Verification items for this drawing (mm, ordinates from the low corner). Coordinates: 2 decimals unless noted, no trailing zeros. Write each loop counter-clockwise with the first axis right and the second up, starting at its lowest first coordinate (ties: lowest second). Pieces come first, ordered by that corner, then holes. Notation, with made-up numbers: M 86,27.25 L 131,27.25 A34 cw 131,58.25 Z; hole C -1,9.5 d10. An arc over 180 degrees is marked long. Put each result on its own line as item: value. Start each with the question number.
1) Gauge pin test, flat ends, axial feed: pin 1 (16 mm diameter, centred on x = 65, y = 90, fed in from -Z); pin 2 (0.8 mm diameter, centred on x = 114, z = 1.5, fed in from +Y). Record the tip position at first contact, or that the pin passes through.
2) Cross-section at B-B on y = 92. Record the cut outline in (x, z).
3) Scan lines: line 1 along Y through (x, z) = (65, 0.7); line 2 along Y through (x, z) = (67, 1.15); line 3 along Y through (x, z) = (6.5, 0.7). Record each from-to range of solid material in increasing order.
4) Cross-section at D-D on x = 89.5. Record the cut outline in (y, z).
5) Cross-section at A-A on x = 65. Record the cut outline in (y, z).
6) Cross-section at C-C on z = 2. Record the cut outline in (x, y), plus the area to 3 significant figures.
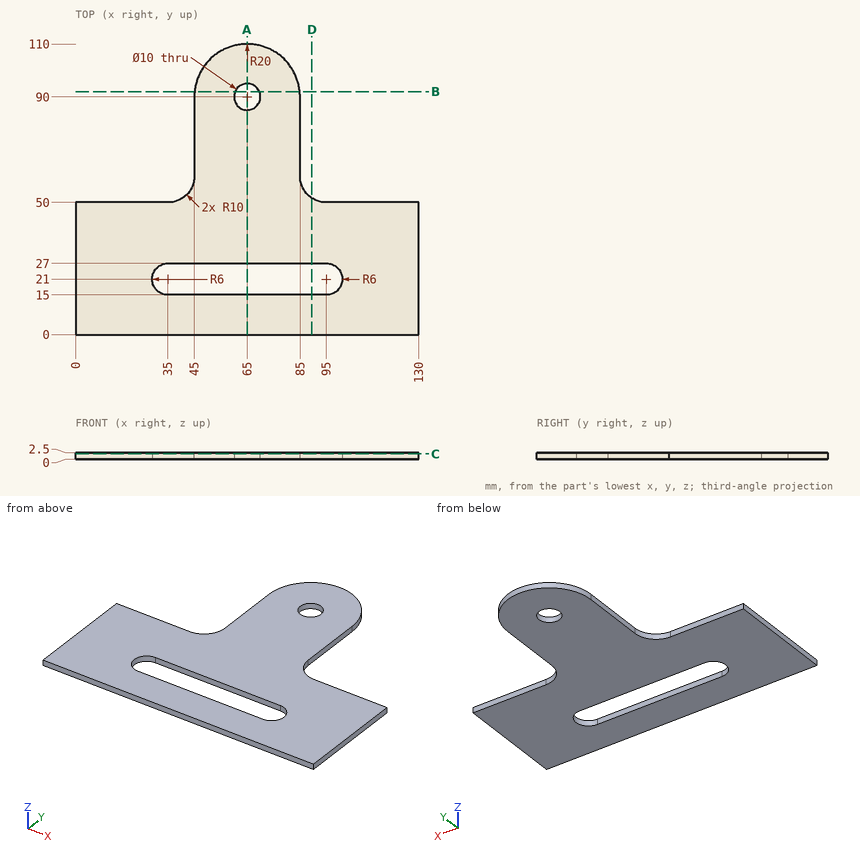
Answer key:
1. pin 1: stops at z = 0
1. pin 2: stops at y = 50
2. outline: M 45.1,0 L 60.42,0 L 60.42,2.5 L 45.1,2.5 Z; M 69.58,0 L 84.9,0 L 84.9,2.5 L 69.58,2.5 Z
3. line 1: y = 0 to 15, 27 to 85, 95 to 110
3. line 2: y = 0 to 15, 27 to 85.42, 94.58 to 109.9
3. line 3: y = 0 to 50
4. outline: M 0,0 L 15,0 L 15,2.5 L 0,2.5 Z; M 27,0 L 51.65,0 L 51.65,2.5 L 27,2.5 Z
5. outline: M 0,0 L 15,0 L 15,2.5 L 0,2.5 Z; M 27,0 L 85,0 L 85,2.5 L 27,2.5 Z; M 95,0 L 110,0 L 110,2.5 L 95,2.5 Z
6. outline: M 0,0 L 130,0 L 130,50 L 95,50 A10 cw 85,60 L 85,90 A20 ccw 45,90 L 45,60 A10 cw 35,50 L 0,50 Z; hole M 35,15 L 95,15 A6 ccw 95,27 L 35,27 A6 ccw Z; hole C 65,90 d10
6. area: 7,860 mm²
